Check sheet for the drawn part. Datum: minimum x, y, z corner. Units: mm. Give positions to 0.01 mm unless a question says otherwise; leave off trailing zeros. Order: outer loops, then holes, each group sorted by start corner. A loop starts at its lowest first (then second) coordinate and runs counter-clockwise, first axis right, second up. Notation, with made-up numbers: (-40, -32.75) -> (-31, -32.75) arc R12 ccw to (-31, -26.75) -> close; hole circle Ø9 at (13.25, 53.25). An arc over 180 degrees is marked (long way). Return JSON: item names as keys, results as strings. Group by question number.
(1) Thickness scan on line 1 along X through (y, z) = (0.25, 28.5); line 2 along X through (y, z) = (0.7, 29.5) (1 decimal); line 3 along Z through (x, y) = (45.5, 3.65). Record the ranges inside material, lowest first.
(2) Cross-section at D-D on x = 8. Enter the section's corners in (y, z) (1 decimal), then the cut area to 3 significant figures.
(3) Cross-section at C-C on x = 18. Enter the section's corners in (y, z).
(4) Depth check by flat-ended pin: pin 1 Ø1.5 at (y, z) = (1.5, 43.5) entering from +X; pin 2 Ø4 at (x, z) = (46.355, 27.305) entering from +Y. Enter the tip coordinate at first touch or a pass-through.
(5) Cross-section at A-A on x = 27. Enter the section's corners in (y, z).
(6) Cross-section at B-B on z = 17.5. Enter the section's corners in (x, y).
(7) Release check for a two-part mould opening along Z. For the marked faces 1 and 2 record: pulls with the +Z half, pulls with the -Z half, needs draft (parallel to the pull), parting line crosses it, or undercut.
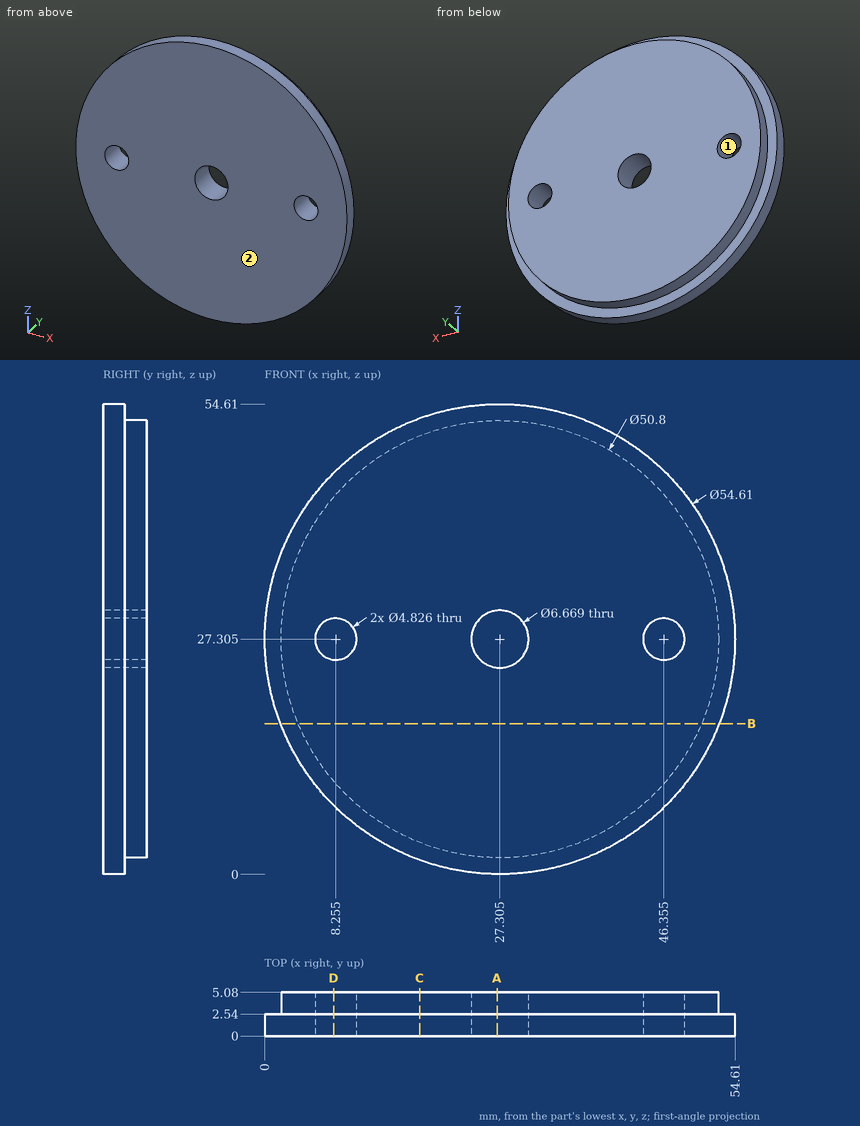
Verdict:
{
 "1": {"line 1": "0.03 to 6.16, 10.35 to 24.19, 30.42 to 44.26, 48.45 to 54.58", "line 2": "0.1 to 7.3, 9.3 to 24.8, 29.8 to 45.4, 47.4 to 54.5", "line 3": "9.58 to 25.05, 29.56 to 45.03"},
 "2": {"outline": "(0, 8) -> (2.5, 8) -> (2.5, 10.8) -> (5.1, 10.8) -> (5.1, 24.9) -> (0, 24.9) -> close; (0, 29.7) -> (5.1, 29.7) -> (5.1, 43.8) -> (2.5, 43.8) -> (2.5, 46.6) -> (0, 46.6) -> close", "area": "158 mm²"},
 "3": {"outline": "(0, 1.63) -> (2.54, 1.63) -> (2.54, 3.67) -> (5.08, 3.67) -> (5.08, 50.94) -> (2.54, 50.94) -> (2.54, 52.98) -> (0, 52.98) -> close"},
 "4": {"pin 1": "x = 49.82", "pin 2": "through"},
 "5": {"outline": "(0, 0) -> (2.54, 0) -> (2.54, 1.91) -> (5.08, 1.91) -> (5.08, 23.98) -> (0, 23.98) -> close; (0, 30.63) -> (5.08, 30.63) -> (5.08, 52.7) -> (2.54, 52.7) -> (2.54, 54.61) -> (0, 54.61) -> close"},
 "6": {"outline": "(1.82, 0) -> (52.79, 0) -> (52.79, 2.54) -> (50.74, 2.54) -> (50.74, 5.08) -> (3.87, 5.08) -> (3.87, 2.54) -> (1.82, 2.54) -> close"},
 "7": {"face 1": "undercut", "face 2": "needs draft"}
}
